from build123d import *

# Parameters (mm, degrees)
SKETCH1_W           = 43
SKETCH1_H           = 40
BOSS_EXTRUDE1_DEPTH = 4
SKETCH2_W           = 43
SKETCH2_H           = 10
BOSS_EXTRUDE2_DEPTH = 45
CUT_EXTRUDE1_REACH  = 68.03
SKETCH3_R           = 12.5
SKETCH3_R_2         = 2


with BuildPart() as part:
    # Sketch1 → Boss-Extrude1 (new body)
    with BuildSketch(Plane(origin=(0, 0, 0), x_dir=(1, 0, 0), z_dir=(0, 1, 0))):
        with Locations((-5.590648476, 5.669439574)):
            Rectangle(SKETCH1_W, SKETCH1_H)
    extrude(amount=BOSS_EXTRUDE1_DEPTH)

    # Sketch2 → Boss-Extrude2 (add)
    with BuildSketch(Plane(origin=(0, 4, 0), x_dir=(1, 0, 0), z_dir=(0, 1, 0))):
        with Locations((-5.590648476, -4.330560426)):
            Rectangle(SKETCH2_W, SKETCH2_H)
    extrude(amount=BOSS_EXTRUDE2_DEPTH)

    # Sketch3 → Cut-Extrude1 (cut, up to next)
    with BuildSketch(Plane.XY.offset(9.330560426), mode=Mode.PRIVATE) as cut_extrude1_sk1:
        with Locations((-5.590648476, 27.5)):
            Circle(SKETCH3_R)
    cut_extrude1_tool1 = extrude(cut_extrude1_sk1.sketch, amount=-CUT_EXTRUDE1_REACH, mode=Mode.PRIVATE) & part.part
    # Sketch3 → Cut-Extrude1 (cut, up to next)
    with BuildSketch(Plane.XY.offset(9.330560426), mode=Mode.PRIVATE) as cut_extrude1_sk2:
        with Locations((-21.090648476, 43)):
            Circle(SKETCH3_R_2)
    cut_extrude1_tool2 = extrude(cut_extrude1_sk2.sketch, amount=-CUT_EXTRUDE1_REACH, mode=Mode.PRIVATE) & part.part
    # Sketch3 → Cut-Extrude1 (cut, up to next)
    with BuildSketch(Plane.XY.offset(9.330560426), mode=Mode.PRIVATE) as cut_extrude1_sk3:
        with Locations((9.909351524, 43)):
            Circle(SKETCH3_R_2)
    cut_extrude1_tool3 = extrude(cut_extrude1_sk3.sketch, amount=-CUT_EXTRUDE1_REACH, mode=Mode.PRIVATE) & part.part
    # Sketch3 → Cut-Extrude1 (cut, up to next)
    with BuildSketch(Plane.XY.offset(9.330560426), mode=Mode.PRIVATE) as cut_extrude1_sk4:
        with Locations((9.909351524, 12)):
            Circle(SKETCH3_R_2)
    cut_extrude1_tool4 = extrude(cut_extrude1_sk4.sketch, amount=-CUT_EXTRUDE1_REACH, mode=Mode.PRIVATE) & part.part
    # Sketch3 → Cut-Extrude1 (cut, up to next)
    with BuildSketch(Plane.XY.offset(9.330560426), mode=Mode.PRIVATE) as cut_extrude1_sk5:
        with Locations((-21.090648476, 12)):
            Circle(SKETCH3_R_2)
    cut_extrude1_tool5 = extrude(cut_extrude1_sk5.sketch, amount=-CUT_EXTRUDE1_REACH, mode=Mode.PRIVATE) & part.part
    add(cut_extrude1_tool1.solids().sort_by_distance((-5.590648, 27.5, 9.33056))[0], mode=Mode.SUBTRACT)
    add(cut_extrude1_tool2.solids().sort_by_distance((-21.090648, 43, 9.33056))[0], mode=Mode.SUBTRACT)
    add(cut_extrude1_tool3.solids().sort_by_distance((9.909352, 43, 9.33056))[0], mode=Mode.SUBTRACT)
    add(cut_extrude1_tool4.solids().sort_by_distance((9.909352, 12, 9.33056))[0], mode=Mode.SUBTRACT)
    add(cut_extrude1_tool5.solids().sort_by_distance((-21.090648, 12, 9.33056))[0], mode=Mode.SUBTRACT)


solid = part.part
The listing builds one solid part. Answer for the finished solid, in the listing's coordinates (mm). A direction names the side the tool comes from. Round coordinates to 2 decimals unless told otherwise and drop trailing zeros. Order: outer loops, then holes, each group sorted by start corner. A loop starts at its lowest first (then second) coordinate and runs counter-clockwise, first axis right, second up. Notation, with made-up numbers: M -40,-4 L -4,-4 A15 ccw -4,12 Z; hole C 43,17.25 d9. An arc over 180 degrees is marked long. Answer in a Markdown table with one row per item. Add a question column.
1) Flat-ended cylindrical pins translate along their axes: pin 1 Ø5 at (x, y) = (-9, 39) entering from -Z; pin 2 Ø6 at (x, y) = (-2.5, 43) entering from +Z; pin 3 Ø4 at (x, z) = (-11, 11.5) entering from +Y. Find the tip coordinate at first contact, or state that the pin passes through.
2) The part is cut by section C-C on x = -0.5. Determine the outline of the cut face in (y, z), plus the area to 3 significant figures.
3) Which of the six approach directions +Z, -Z, +X, -X, +Y, -Y give full straight-line access (tool end or side, diameter ignored) to faces 5 (the face through (-6, 0, -6)), 6 (the face through (-6, 4, 12)), 7 (the face through (-6, 4, -13))?
4) Consider line 1 along X through (y, z) = (27, 4); line 2 along Z through (x, y) = (-2, 14.5); line 3 along Y through (x, z) = (12, -4). Determine where each line is inside the solid, lowest interval first. Write a range as from..to.
5) The part is cut by section A-A on z = 5. Determine the outline of the cut face in (x, y).
6) The part is cut by section D-D on y = 27.5. Determine the outline of the cut face in (x, z).
7) Determine the mould class of faces 1 (the face through (9.476, 41.048, 4.401)), 2 (the face through (-15, 36, -0.669)), 3 (the face through (-21.524, 41.048, 4.401)), 4 (the face through (-27.091, 21, 2)) for opening direction X: pulls with the +X half, pulls with the -X half, needs draft (parallel to the pull), parting line crosses it, or undercut.
8) The part is cut by section B-B on y = 12. Determine the outline of the cut face in (x, z), plus the area to 3 significant figures.
Findings below:
| question | item | result |
|---|---|---|
| 1 | pin 1 | stops at z = -0.67 |
| 1 | pin 2 | stops at z = 9.33 |
| 1 | pin 3 | stops at y = 4 |
| 2 | outline | M 0,-25.67 L 4,-25.67 L 4,-0.67 L 16.08,-0.67 L 16.08,9.33 L 4,9.33 L 4,14.33 L 0,14.33 Z; M 38.92,-0.67 L 49,-0.67 L 49,9.33 L 38.92,9.33 Z |
| 2 | area | 382 mm² |
| 3 | face 5 | +Z, -Z, +X, -X, -Y |
| 3 | face 6 | +Z, +X, -X, +Y |
| 3 | face 7 | -Z, +X, -X, +Y |
| 4 | line 1 | x = -27.09..-18.08, 6.9..15.91 |
| 4 | line 2 | z = -0.67..9.33 |
| 4 | line 3 | y = 0..4 |
| 5 | outline | M -27.09,0 L 15.91,0 L 15.91,49 L -27.09,49 Z; hole C -21.09,12 d4; hole C -21.09,43 d4; hole C -5.59,27.5 d25; hole C 9.91,12 d4; hole C 9.91,43 d4 |
| 6 | outline | M -27.09,-0.67 L -18.09,-0.67 L -18.09,9.33 L -27.09,9.33 Z; M 6.91,-0.67 L 15.91,-0.67 L 15.91,9.33 L 6.91,9.33 Z |
| 7 | face 1 | undercut |
| 7 | face 2 | needs draft |
| 7 | face 3 | undercut |
| 7 | face 4 | pulls with the -X half |
| 8 | outline | M -27.09,-0.67 L -23.09,-0.67 L -23.09,9.33 L -27.09,9.33 Z; M -19.09,-0.67 L 7.91,-0.67 L 7.91,9.33 L -19.09,9.33 Z; M 11.91,-0.67 L 15.91,-0.67 L 15.91,9.33 L 11.91,9.33 Z |
| 8 | area | 350 mm² |
